Autodesk Inventor part; units mm, degrees
ref_plane "YZ Plane" through (0, 0, 0) normal (1, 0, 0) x (0, 1, 0)
ref_plane "XZ Plane" through (0, 0, 0) normal (0, 1, 0) x (-1, 0, 0)
ref_plane "XY Plane" through (0, 0, 0) normal (0, 0, 1) x (1, 0, 0)
sketch "Sketch1" plane through (0, 0, 0) normal (0, 0, 1) x (1, 0, 0)
  line L0 (0, 0) -> (850.9, 0)
  line L1 (850.9, 0) -> (850.9, 76.2)
  line L2 (850.9, 76.2) -> (0, 76.2)
  line L3 (0, 76.2) -> (0, 0)
  dimension "d0" = 850.9
  dimension "d1" = 76.2
extrude "Extrusion1" add sketch "Sketch1" along normal blind 3.175
sketch "Sketch2" plane through (0, 0, 3.175) normal (0, 0, 1) x (1, 0, 0)
  line L0 (0, 0) -> (850.9, 0)
  circle A0 centre (292.9509, 36.5125) radius 14.2875
  circle A1 centre (557.9491, 36.5125) radius 14.2875
  circle A2 centre (92.9313, 39.6875) radius 14.2875
  circle A3 centre (757.9235, 39.6875) radius 14.2875
  line L1 (0, 0) -> (25.4, 0)
  line L2 (0, 0) -> (0, 38.1)
  line L3 (0, 76.2) -> (0, 0)
  line L4 (0, 38.1) -> (25.4, 0)
  circle A4 centre (34.925, 12.7) radius 3.5687
  circle A5 centre (12.7, 66.675) radius 3.5687
  line L5 (850.9, 76.2) -> (0, 76.2)
  line L6 (850.9, 0) -> (850.9, 38.1)
  line L7 (850.9, 0) -> (850.9, 76.2)
  line L8 (850.9, 0) -> (825.5, 0)
  line L9 (825.5, 0) -> (850.9, 38.1)
  circle A6 centre (190.5, 38.1) radius 3.5687
  line L10 (825.5, 0) -> (800.1, 0)
  circle A7 centre (815.975, 12.7) radius 3.5687
  circle A8 centre (831.85, 57.15) radius 3.5687
  circle A9 centre (425.45, 66.675) radius 3.5687
  circle A10 centre (425.45, 9.525) radius 3.5687
  circle A11 centre (190.5, 9.525) radius 3.5687
  circle A12 centre (190.5, 66.675) radius 3.5687
  circle A13 centre (660.4, 66.675) radius 3.5687
  circle A14 centre (660.4, 9.525) radius 3.5687
  dimension "d10" = 28.575
  dimension "d23" = 28.575
  dimension "d30" = 28.575
  dimension "d32" = 28.575
  dimension "d34" = 25.4
  dimension "d35" = 38.1
  dimension "d36" = 7.1374
  dimension "d37" = 12.7
  dimension "d38" = 9.525
  dimension "d40" = 7.1374
  dimension "d41" = 12.7
  dimension "d42" = 9.525
  dimension "d43" = 38.1
  dimension "d44" = 25.4
  dimension "d53" = 7.1374
  dimension "d54" = 38.1
  dimension "d55" = 190.5
  dimension "d59" = 7.1374
  dimension "d60" = 12.7
  dimension "d61" = 9.525
  dimension "d66" = 7.1374
  dimension "d67" = 7.1374
  dimension "d68" = 9.525
  dimension "d69" = 425.45
  dimension "d70" = 7.1374
  dimension "d71" = 9.525
  dimension "d72" = 425.45
  dimension "d73" = 7.1374
  dimension "d74" = 7.1374
  dimension "d75" = 9.525
  dimension "d76" = 9.525
  dimension "d77" = 190.5
  dimension "d78" = 190.5
  dimension "d79" = 7.1374
  dimension "d80" = 7.1374
  dimension "d81" = 9.525
  dimension "d82" = 9.525
  dimension "d83" = 190.5
  dimension "d84" = 190.5
extrude "Extrusion2" cut sketch "Sketch2" against normal blind 3.175 contours L2 L4 L0 | L9 L6 L0 | A0 | A1 | A2 | A3 | A4 | A5 | A6 | A7 | A8 | A9 | A10 | A11 | A12 | A13 | A14
sketch "Sketch3" plane through (0, 0, 3.175) normal (0, 0, 1) x (1, 0, 0)
  circle A0 centre (190.5, 38.1) radius 3.5687
  circle A1 centre (831.85, 57.15) radius 3.5687
  line L0 (179.2605, 25.273) -> (201.7395, 25.273)
  line L1 (203.327, 26.8605) -> (203.327, 49.3395)
  line L2 (201.7395, 50.927) -> (179.2605, 50.927)
  line L3 (177.673, 49.3395) -> (177.673, 26.8605)
  line L4 (177.673, 25.273) -> (203.327, 50.927) construction
  line L5 (203.327, 25.273) -> (177.673, 50.927) construction
  line L6 (843.0895, 44.323) -> (820.6105, 44.323)
  line L7 (819.023, 45.9105) -> (819.023, 68.3895)
  line L8 (820.6105, 69.977) -> (843.0895, 69.977)
  line L9 (844.677, 68.3895) -> (844.677, 45.9105)
  line L10 (844.677, 44.323) -> (819.023, 69.977) construction
  line L11 (819.023, 44.323) -> (844.677, 69.977) construction
  circle A2 centre (581.7616, 36.5125) radius 2.8067
  circle A3 centre (534.1366, 36.5125) radius 2.8067
  circle A4 centre (500.7991, 36.5125) radius 2.8067
  circle A5 centre (615.0991, 36.5125) radius 2.8067
  arc A6 (179.2605, 50.927) -> (177.673, 49.3395) centre (179.2605, 49.3395) ccw
  arc A7 (203.327, 49.3395) -> (201.7395, 50.927) centre (201.7395, 49.3395) ccw
  arc A8 (201.7395, 25.273) -> (203.327, 26.8605) centre (201.7395, 26.8605) ccw
  arc A9 (177.673, 26.8605) -> (179.2605, 25.273) centre (179.2605, 26.8605) ccw
  arc A10 (820.6105, 69.977) -> (819.023, 68.3895) centre (820.6105, 68.3895) ccw
  arc A11 (844.677, 68.3895) -> (843.0895, 69.977) centre (843.0895, 68.3895) ccw
  arc A12 (843.0895, 44.323) -> (844.677, 45.9105) centre (843.0895, 45.9105) ccw
  arc A13 (819.023, 45.9105) -> (820.6105, 44.323) centre (820.6105, 45.9105) ccw
  point P0 (0, 0)
  dimension "d88" = 25.654
  dimension "d89" = 25.654
  dimension "d90" = 25.654
  dimension "d91" = 25.654
  dimension "d93" = 5.6134
  dimension "d94" = 5.6134
  dimension "d96" = 5.6134
  dimension "d97" = 5.6134
  dimension "d98" = 1.5875
extrude "Extrusion4" cut sketch "Sketch3" against normal blind 25.4
properties part number "InsidePlate" material "Aluminum 6061"
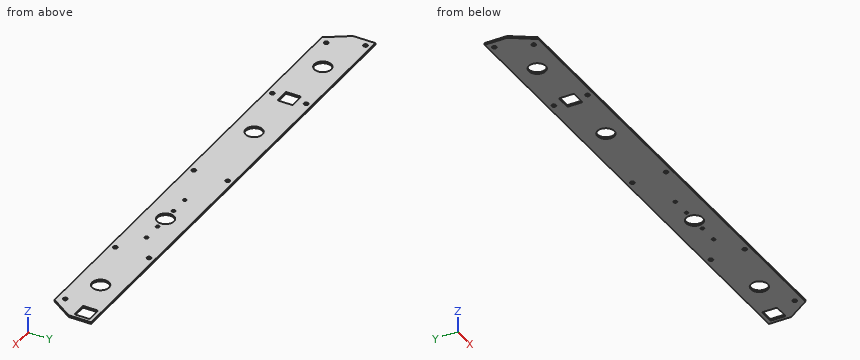
Model file for the job. Use its own axes, mm. Coordinates: 2 decimals unless noted, no trailing zeros. Return JSON: item names as keys, results as strings. Group by question number.
Item 1: Flat gauge pins, fed straight in: P1, Ø1, axis at x = 837.5, z = 1.5, coming from the -Y side; P2, Ø1, axis at y = 24.5, z = 2, coming from the +X side. Where does each tip first touch, or does it go through?
Item 2: Saw through at A-A on z = 1.15. State how many separate pieces and enclosed holes the cut face has, then the cut area to 3 significant figures.
Item 3: Wall check: line 1 along X through (y, z) = (66.5, 0.75); line 2 along X through (y, z) = (67.5, 0.95); line 3 along Y through (x, z) = (190.5, 2.2). Give the ranges that are in metal, low to high. Write a range as [from, to].
Values found:
{
 "1": {"P1": "stops at y = 17.25", "P2": "stops at x = 842.17"},
 "2": {"separate pieces": "1", "enclosed holes": "19", "area": "59,500 mm2"},
 "3": {"line 1": "x = [0, 9.14], [16.26, 186.94], [194.06, 421.89], [429.01, 656.84], [663.96, 819.02], [844.68, 850.9]", "line 2": "x = [0, 9.23], [16.17, 187.03], [193.97, 421.98], [428.92, 656.93], [663.87, 819.02], [844.68, 850.9]", "line 3": "y = [0, 5.96], [13.09, 25.27], [50.93, 63.11], [70.24, 76.2]"}
}
